```python
from build123d import *

# Parameters (mm, degrees)
F1_DEPTH = 25.4
F2_R     = 2.54


with BuildPart() as f1:
    # F0 (on Top) → F1 (new body)
    with BuildSketch(Plane.XY):
        Polygon((24.431467, 13.838641), (-30.526407, 13.838641), (-30.526407, 0), (-30.526407, -12.888923), (24.431467, -12.810618), align=None)
    extrude(amount=F1_DEPTH)

    # F2
    f2_edges = [f1.edges().sort_by_distance(p)[0] for p in [
        (-3.04747, -12.84977, 25.4),
        (-3.04747, 13.838641, 25.4),
        (24.431467, 0.514012, 25.4),
        (-30.526407, 0.474859, 25.4),
    ]]
    fillet(f2_edges, radius=F2_R)


solid = f1.part
```
Input: part model. Units: mm. Frame: model coordinates. A direction names the side the tool comes from. Coordinates: 2 decimals unless noted, no trailing zeros. Use one line per item in the form item = value.
Q1. First-contact query: pin 1 (8 mm diameter, centred on x = -7.5, y = 9, fed in from -Z). Flat tip, straight axial feed; report the tip coordinate or a pass-through.
Answer below:
pin_1 = 0
Q2. Material intervals for probe 1 along Y at (x, z) = (-6.5, 13); probe 2 along Y at (x, z) = (-5, 24); probe 3 along Z at (x, y) = (8, -11.5), sorted ascending. Write a range as from..to.
Answer below:
probe_1 = -12.85..13.84
probe_2 = -12.58..13.57
probe_3 = 0..25.1
Q3. Set-up query: faces 1 (the face through (-3, 1, 25.4)), 2 (the face through (-2.66, -12.12, 24.64)). Return all of +Z, -Z, +X, -X, +Y, -Y with unobstructed straight access to the full face (end or side cutting, diameter ignored); none if empty.
Answer below:
face_1 = +Z, +X, -X, +Y, -Y
face_2 = +Z, +X, -Y
